Design review of the part built by this model. Coordinates are the model's own, in mm. A direction names the side the tool comes from. Coordinates: 2 decimals unless noted, no trailing zeros. Write each loop counter-clockwise with the first axis right and the second up, starting at its lowest first coordinate (ties: lowest second). Pieces come first, ordered by that corner, then holes. Notation, with made-up numbers: M 1,52.5 L 10,52.5 A31 cw 10,90.5 Z; hole C 40.5,34 d10. An arc over 180 degrees is marked long. Return JSON: item names as keys, results as strings. Group by question number.
```python
from build123d import *

# Parameters (mm, degrees)
F0_W     = 1200
F0_H     = 600
F1_DEPTH = 250
F2_W     = 200
F2_H     = 250
F3_DEPTH = 250.001
F5_DEPTH = 250
F6_R     = 110
F7_DEPTH = 500.001
F9_DEPTH = 600.001


with BuildPart() as f1:
    # F0 (on Top) → F1 (new body)
    with BuildSketch(Plane.XY):
        Rectangle(F0_W, F0_H)
    extrude(amount=F1_DEPTH)

    # F2 (on face) → F3 (cut, through all)
    with BuildSketch(Plane.XY.offset(250)):
        with Locations((-500, 0)):
            Rectangle(F2_W, F2_H)
        with Locations((500, 0)):
            Rectangle(F2_W, F2_H)
    extrude(amount=-F3_DEPTH, mode=Mode.SUBTRACT)

    # F4 (on face) → F5 (join)
    with BuildSketch(Plane.XY.offset(250)):
        Polygon((-300, 0), (0, -300), (300, 0), (0, 300), align=None)
    extrude(amount=F5_DEPTH)

    # F6 (on face) → F7 (cut, through all)
    with BuildSketch(Plane.XY.offset(500)):
        Circle(F6_R)
    extrude(amount=-F7_DEPTH, mode=Mode.SUBTRACT)

    # F8 (on face) → F9 (cut, through all)
    with BuildSketch(Plane.XZ.offset(300)):
        with BuildLine():
            Line((-90, 0), (90, 0))
            ThreePointArc((90, 0), (0, 90), (-90, 0))
        make_face()
    extrude(amount=-F9_DEPTH, mode=Mode.SUBTRACT)


solid = f1.part
```
Item 1: Machinability: for faces 4 (the flat face through (-152, -148, 373)), 5 (the flat face through (152, 148, 373)), 6 (the flat face through (362, 4, 250)), 7 (the flat face through (-148, 152, 373)), 8 (the flat face through (-501, -125, 127)), which of the approach directions +Z, -Z, +X, -X, +Y, -Y give a long, thin tool a straight path to every point of the face, cutting with its end or side? Answer none if there is none.
Item 2: Add section B-B (x = -22). Write out the cut boundary in (y, z).
Item 3: For line 1 (X direction, y = 0, z = 103); line 2 (X direction, y = 0, z = 370); line 3 (Y direction, x = 533, z = 131), list the stretches that pass through material, from the lowest coordinate up.
Item 4: Add section C-C (x = 207.5). Write out the cut boundary in (y, z).
Item 5: Add section D-D (y = -151.5). Write out the cut boundary in (x, z).
Item 6: For pin 1 (12 mm diameter, centred on y = 26, z = 374, fed in from +X); pin 2 (8 mm diameter, centred on x = 287, z = 373, fed in from -Y); pin 3 (3 mm diameter, centred on x = 128.5, z = 398.5, fed in from -Y), all flat-tipped, find the tip position at first contact; note any pin that passes through.
Item 7: The part is to be moulded in two halves that separate along Y. For faces 1 (the flat face through (600, 211, 123)), 2 (the flat face through (-8, -300, 123)), 3 (the flat face through (400, -2, 127)), say which applies: pulls with the +Y half, pulls with the -Y half, needs draft (parallel to the pull), parting line crosses it, or undercut.
Item 8: Add section A-A (z = 177.5). Write out the cut boundary in (x, y).
Geometry check:
{
 "1": {"face 4": "+Z, -X, -Y", "face 5": "+Z, +X, +Y", "face 6": "+Z, +X", "face 7": "+Z, -X, +Y", "face 8": "+Z, -Z, -X"},
 "2": {"outline": "M -300,87.27 L -107.78,87.27 L -107.78,500 L -278,500 L -278,250 L -300,250 Z; M 107.78,87.27 L 300,87.27 L 300,250 L 278,250 L 278,500 L 107.78,500 Z"},
 "3": {"line 1": "-400 to -110, 110 to 400", "line 2": "-300 to -110, 110 to 300", "line 3": "-300 to -125, 125 to 300"},
 "4": {"outline": "M -300,0 L 300,0 L 300,250 L 92.5,250 L 92.5,500 L -92.5,500 L -92.5,250 L -300,250 Z"},
 "5": {"outline": "M -600,0 L -90,0 A90 cw 90,0 L 600,0 L 600,250 L 148.5,250 L 148.5,500 L -148.5,500 L -148.5,250 L -600,250 Z"},
 "6": {"pin 1": "x = 280", "pin 2": "y = -17", "pin 3": "y = -173"},
 "7": {"face 1": "needs draft", "face 2": "pulls with the -Y half", "face 3": "undercut"},
 "8": {"outline": "M -600,-300 L 600,-300 L 600,-125 L 400,-125 L 400,125 L 600,125 L 600,300 L -600,300 L -600,125 L -400,125 L -400,-125 L -600,-125 Z; hole C 0,0 d220"}
}
